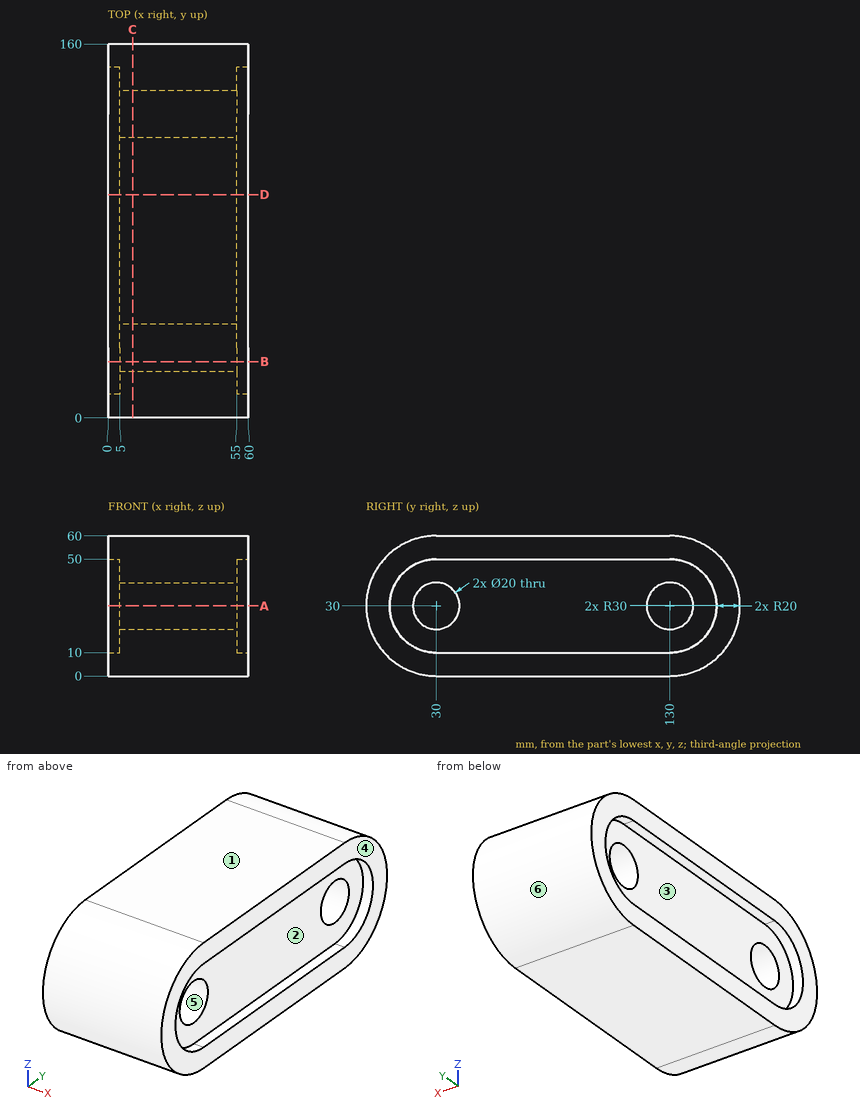
Check sheet for the drawn part. Datum: minimum x, y, z corner. Units: mm. A direction names the side the tool comes from. Give positions to 0.01 mm unless a question says otherwise; leave off trailing zeros. Write each loop counter-clockwise with the first axis right and the second up, starting at its lowest first coordinate (ties: lowest second). Pieces come first, ordered by that corner, then holes. Notation, with made-up numbers: M -4,50.5 L 11,50.5 A31 ccw 11,74.5 Z; hole C 21.25,68 d2. An arc over 180 degrees is marked long. Write item = value, one per line.
(1) Sectioned sample at D-D (y = 95.5). Record the cut outline in (x, z).
Found:
outline = M 0,0 L 60,0 L 60,10 L 55,10 L 55,50 L 60,50 L 60,60 L 0,60 L 0,50 L 5,50 L 5,10 L 0,10 Z
(2) Sectioned sample at C-C (x = 10.5). Record the cut outline in (y, z).
Found:
outline = M 30,0 L 130,0 A30 ccw 130,60 L 30,60 A30 ccw Z; hole C 30,30 d20; hole C 130,30 d20
(3) Draft check along Z on the marked faces 3, 4, 5 and 6. Enter one of: released by +Z, released by -Z, zero draft, split by the parting line, or undercut.
Found:
face_3 = undercut
face_4 = zero draft
face_5 = undercut
face_6 = split by the parting line
(4) Go/stop test with flat-tipped pins: pin 1 Ø12 at (y, z) = (30, 30) entering from +X; pin 2 Ø10 at (x, z) = (22.5, 29) entering from -Y; pin 3 Ø3 at (y, z) = (26, 15) entering from -X; pin 4 Ø6 at (x, z) = (49.5, 21) entering from -Y. Record where each tip stops, or that it passes through.
Found:
pin_1 = through
pin_2 = 0
pin_3 = 5
pin_4 = 0.61
(5) Material ranges on line 1 (Y direction, x = 37, z = 37); line 2 (Z direction, x = 44, y = 30); line 3 (Y direction, x = 37.5, z = 24), recorded low to high.
Found:
line_1 = 0.83 to 22.86, 37.14 to 122.86, 137.14 to 159.17
line_2 = 0 to 20, 40 to 60
line_3 = 0.61 to 22, 38 to 122, 138 to 159.39
(6) Sectioned sample at B-B (y = 24). Record the cut outline in (x, z), then the cut area to 3 significant figures.
Found:
outline = M 0,0.61 L 60,0.61 L 60,10.92 L 55,10.92 L 55,22 L 5,22 L 5,10.92 L 0,10.92 Z; M 0,49.08 L 5,49.08 L 5,38 L 55,38 L 55,49.08 L 60,49.08 L 60,59.39 L 0,59.39 Z
area = 2,350 mm2
(7) Sectioned sample at A-A (z = 30). Record the cut outline in (x, y).
Found:
outline = M 0,0 L 60,0 L 60,10 L 55,10 L 55,20 L 5,20 L 5,10 L 0,10 Z; M 0,150 L 5,150 L 5,140 L 55,140 L 55,150 L 60,150 L 60,160 L 0,160 Z; M 5,40 L 55,40 L 55,120 L 5,120 Z
(8) Access from +Z, -Z, +X, -X, +Y, -Y to the whole of each face (thin tool, end or side, straight path). Record for the marked faces 1 and 2.
Found:
face_1 = +Z, +X, -X, +Y, -Y
face_2 = +X
